from build123d import *

# Parameters (mm, degrees)
F0_W     = 88.6754395919
F0_H     = 62.5690418352
F0_R     = 5.588
F1_DEPTH = 25.4
F2_DEPTH = 6.35
F3_DEPTH = 25.4
F4_DEPTH = 10.06593


with BuildPart() as f1:
    # F0 (on Front) → F1 (new body)
    with BuildSketch(Plane.XZ):
        with Locations((4.6873632818, 2.5576064363)):
            Rectangle(F0_W, F0_H)
        with Locations((-19.05, 0)):
            Circle(F0_R, mode=Mode.SUBTRACT)
        with Locations((19.05, 0.2921762194)):
            Circle(F0_R, mode=Mode.SUBTRACT)
        with Locations((-19.05, 0)):
            Circle(F0_R)
        with Locations((19.05, 0.2921762194)):
            Circle(F0_R)
    extrude(amount=F1_DEPTH)

    # F0 (on Front) → F2 (join)
    with BuildSketch(Plane.XZ):
        with Locations((19.05, 0.2921762194)):
            Circle(F0_R)
        with Locations((-19.05, 0)):
            Circle(F0_R)
    extrude(amount=-F2_DEPTH)

    # F3 (add): a face of the model
    f3_faces = [f1.faces().sort_by_distance(p)[0] for p in [
        (-39.6503565141, -12.7, 2.5576064363),
    ]]
    extrude(f3_faces, amount=F3_DEPTH)

    # F4 (add): a face of the model
    f4_faces = [f1.faces().sort_by_distance(p)[0] for p in [
        (49.0250830778, -12.7, 2.5576064363),
    ]]
    extrude(f4_faces, amount=F4_DEPTH)


solid = f1.part
Could you check a few things on this model? Use its own coordinates, in mm. Give positions to 0.01 mm unless a question says otherwise; leave off trailing zeros. Order: outer loops, then holes, each group sorted by start corner. A loop starts at its lowest first (then second) coordinate and runs counter-clockwise, first axis right, second up. Notation, with made-up numbers: (-35, -11.5) -> (17, -11.5) arc R24 cw to (17, 22.5) -> close; hole circle Ø11 at (78, 40.25). An arc over 180 degrees is marked (long way). Answer in a Markdown table with one row per item. Add a question column.
Item 1: We'd pull the mould along X, two halves only. Please class faces 1 (the flat face through (59.091, -13, 2)), 2 (the flat face through (-4, -13, -28.727)), 3 (the cylindrical face through (13.467, 3.131, 0.538)), 4 (the cylindrical face through (-23.484, 3.131, -3.4)): pulls with the +X half, pulls with the -X half, needs draft (parallel to the pull), parting line crosses it, or undercut.
Item 2: Imagine slicing it at A-A (x = 19.05). List the corners of the cut face in (y, z) for me.
Item 3: Please list where these lines run through material, in increasing order: probe 1 along Y at (x, z) = (-46.5, 14); probe 2 along X at (y, z) = (1.5, 4).
Item 4: Imagine slicing it at B-B (z = -3). List the corners of the cut face in (x, y) for me, and give its area (3 significant figures).
Item 5: Imagine slicing it at D-D (z = 27.5). List the corners of the cut face in (x, y) for me.
Item 6: I'm going to push a flat-ended pin straight in: P1, Ø5, axis at x = -46, z = -7.5, coming from the +Y side. Where does the tip first touch, or does it pass through?
Item 7: Imagine slicing it at C-C (y = 2.5). List the corners of the cut face in (x, z) for me.
Result:
| question | item | result |
|---|---|---|
| 1 | face 1 | pulls with the +X half |
| 1 | face 2 | needs draft |
| 1 | face 3 | undercut |
| 1 | face 4 | undercut |
| 2 | outline | (-25.4, -28.73) -> (0, -28.73) -> (0, -5.3) -> (6.35, -5.3) -> (6.35, 5.88) -> (0, 5.88) -> (0, 33.84) -> (-25.4, 33.84) -> close |
| 3 | probe 1 | -25.4 to 0 |
| 3 | probe 2 | -22.95 to -15.15, 14.87 to 23.23 |
| 4 | outline | (-65.05, -25.4) -> (59.09, -25.4) -> (59.09, 0) -> (23.57, 0) -> (23.57, 6.35) -> (14.53, 6.35) -> (14.53, 0) -> (-14.34, 0) -> (-14.34, 6.35) -> (-23.76, 6.35) -> (-23.76, 0) -> (-65.05, 0) -> close |
| 4 | area | 3,270 mm2 |
| 5 | outline | (-65.05, -25.4) -> (59.09, -25.4) -> (59.09, 0) -> (-65.05, 0) -> close |
| 6 | P1 | y = 0 |
| 7 | outline | circle Ø11.18 at (-19.05, 0); circle Ø11.18 at (19.05, 0.29) |
